Work out the finished part from the listing and answer in its coordinate system (mm). Face numbers are marked on the shaded views. A direction names the side the tool comes from. Coordinates: 2 decimals unless noted, no trailing zeros. Write each loop counter-clockwise with the first axis right and the second up, starting at its lowest first coordinate (ties: lowest second). Pieces come first, ordered by that corner, then holes. Notation, with made-up numbers: (59, 16.5) - (111, 16.5) arc R28 cw to (111, 53.5) - close; hole circle Ø2 at (1.5, -33). An arc over 180 degrees is marked (long way). Use a Markdown table: item, result. Add a question column.
(1) For a pull along Y with two mould halves and no side action, classify the marked faces 6, 7, 8 and 9 as released by +Y, released by -Y, zero draft, split by the parting line, or undercut.
(2) The part is cut by section C-C, the plane y = -9.5. Give the vertices of the cut face in (x, z).
(3) The part is cut by section B-B, the plane x = 0. Give the vertices of the cut face in (y, z), then the cut area to 3 significant figures.
(4) A tool of negligible diameter and unlimited length cuts with its end or side. For the marked faces 1, 2, 3, 4 and 5, from which of +Z, -Z, +X, -X, +Y, -Y can it reach the whole face along a straight path? Write none if from no direction.
(5) The part is cut by section A-A, the plane y = -37. Give the vertices of the cut face in (x, z).
(6) Find the intervals of material crossed by line 1 (Y direction, x = 0, z = 2.25); line 2 (X direction, y = -57, z = 3); line 3 (Y direction, x = 19, z = 7.5), in increasing order. Write a range as from..to.
(7) The part is cut by section D-D, the plane z = 4.25. Give the vertices of the cut face in (x, y).
(8) Given pin 1 Ø10 at (x, y) = (-1, -83) entering from +Z; pin 2 Ø2 at (x, z) = (-22, 3.5) entering from -Y; pin 3 Ø2 at (y, z) = (-29, 8) entering from +X; pin 4 Ø10 at (x, y) = (-3, -54) entering from -Z, each flat-ended and moving along its own axis, determine where each tip first touches the part or whether it passes through.
from build123d import *

# Parameters (mm, degrees)
SKETCH2_R           = 5.08
BOSS_EXTRUDE1_DEPTH = 8.89
CUT_EXTRUDE1_DEPTH  = 8.89
CUT_EXTRUDE4_DEPTH  = 1.778
CUT_EXTRUDE5_START  = -1.778
CUT_EXTRUDE5_DEPTH  = 1.778
SKETCH13_W          = 8.89
SKETCH13_H          = 6.560107066
BOSS_EXTRUDE6_DEPTH = 7.62
SKETCH14_W          = 8.89
SKETCH14_H          = 6.560107066
BOSS_EXTRUDE7_DEPTH = 7.62
FILLET1_R           = 2.032
SKETCH15_R          = 3.556
CUT_EXTRUDE6_DEPTH  = 3.81


with BuildPart() as part:
    # Sketch2 → Boss-Extrude1 (new body)
    with BuildSketch(Plane.XY):
        with BuildLine():
            Line((-10.406791551, -8.202588674), (-10.406791551, -66.622588674))
            ThreePointArc((-10.406791551, -66.622588674), (-12.510019722, -78.309204867), (-18.555768436, -88.529258158))
            Line((-18.555768436, -88.529258158), (-18.555768436, -95.089365224))
            Line((-18.555768436, -95.089365224), (18.555768436, -95.089365224))
            Line((18.555768436, -95.089365224), (18.555768436, -88.529258158))
            ThreePointArc((18.555768436, -88.529258158), (12.510019722, -78.309204867), (10.406791551, -66.622588674))
            Line((10.406791551, -66.622588674), (10.406791551, -8.202588674))
            ThreePointArc((10.406791551, -8.202588674), (0, 0), (-10.406791551, -8.202588674))
        make_face()
        with Locations((0, -10.702948686)):
            Circle(SKETCH2_R, mode=Mode.SUBTRACT)
    extrude(amount=BOSS_EXTRUDE1_DEPTH)

    # Sketch3 → Cut-Extrude1 (cut)
    with BuildSketch(Plane.XY.offset(8.89)):
        with BuildLine():
            Line((-15.392321471, -95.089365224), (15.087678529, -95.089365224))
            ThreePointArc((15.087678529, -95.089365224), (-0.152321471, -79.849365224), (-15.392321471, -95.089365224))
        make_face()
    extrude(amount=-CUT_EXTRUDE1_DEPTH, mode=Mode.SUBTRACT)

    # Sketch8 → Cut-Extrude4 (cut)
    with BuildSketch(Plane.XY.offset(8.89)):
        with BuildLine():
            Line((-6.35, -32.367098726), (-6.35, -57.618798646))
            ThreePointArc((-6.35, -57.618798646), (0, -63.968798646), (6.35, -57.618798646))
            Line((6.35, -57.618798646), (6.35, -32.367098726))
            ThreePointArc((6.35, -32.367098726), (0, -26.017098726), (-6.35, -32.367098726))
        make_face()
    extrude(amount=-CUT_EXTRUDE4_DEPTH, mode=Mode.SUBTRACT)

    # Sketch9 → Cut-Extrude5 (cut)
    with BuildSketch(Plane(origin=(0, 0, 0), x_dir=(-1, 0, 0), z_dir=(0, 0, -1)).offset(CUT_EXTRUDE5_START)):
        with BuildLine():
            Line((6.35, -57.618798646), (6.35, -32.367098726))
            ThreePointArc((6.35, -32.367098726), (0, -26.017098726), (-6.35, -32.367098726))
            Line((-6.35, -32.367098726), (-6.35, -57.618798646))
            ThreePointArc((-6.35, -57.618798646), (0, -63.968798646), (6.35, -57.618798646))
        make_face()
    extrude(amount=CUT_EXTRUDE5_DEPTH, mode=Mode.SUBTRACT)

    # Sketch13 → Boss-Extrude6 (add)
    with BuildSketch(Plane.ZY.offset(18.555768436)):
        with Locations((4.445, -91.809311691)):
            Rectangle(SKETCH13_W, SKETCH13_H)
    extrude(amount=BOSS_EXTRUDE6_DEPTH)

    # Sketch14 → Boss-Extrude7 (add)
    with BuildSketch(Plane(origin=(18.555768436, 0, 0), x_dir=(0, 0, -1), z_dir=(1, 0, 0))):
        with Locations((-4.445, -91.809311691)):
            Rectangle(SKETCH14_W, SKETCH14_H)
    extrude(amount=BOSS_EXTRUDE7_DEPTH)

    # Fillet1
    # the kernel refuses this fillet: 2.032 mm, written as the material it takes off along each edge
    with BuildSketch(Plane(origin=(0, -57.618798646, 0), x_dir=(1, 0, 0), z_dir=(0, 1, 0))) as fillet1_piece_1:
        with BuildLine():
            CenterArc((8.366062499, -2.032), FILLET1_R, 90, 82.819244219)
            Line((6.35, -1.778), (6.30967875, -1.77292))
            ThreePointArc((6.30967875, -1.77292), (6.30936, -0.889), (6.30936, 0))
            Line((6.30936, 0), (6.35, 0.04064))
            Line((6.35, 0.04064), (8.366062499, 0.04064))
            Line((8.366062499, 0.04064), (8.366062499, 0))
        make_face()
    revolve(axis=Axis((0, -57.618798646, 0), (0, 0, -1)), revolution_arc=180, mode=Mode.SUBTRACT)
    with BuildSketch(Plane(origin=(-6.35, -57.618798646, 0), x_dir=(-1, 0, 0), z_dir=(0, 1, 0)), Plane(origin=(6.35, -32.367098726, 0), x_dir=(1, 0, 0), z_dir=(0, -1, 0)), Plane(origin=(-6.35, -32.367098726, 8.89), x_dir=(-1, 0, 0), z_dir=(0, -1, 0)), Plane(origin=(6.35, -57.618798646, 8.89), x_dir=(1, 0, 0), z_dir=(0, 1, 0))) as fillet1_piece_2:
        with BuildLine():
            CenterArc((2.016062499, 2.032), FILLET1_R, 187.180755781, 82.819244219)
            Line((0, 1.778), (-0.04032125, 1.77292))
            ThreePointArc((-0.04032125, 1.77292), (-0.04064, 0.889), (-0.04064, 0))
            Line((-0.04064, 0), (0, -0.04064))
            Line((0, -0.04064), (2.016062499, -0.04064))
            Line((2.016062499, -0.04064), (2.016062499, 0))
        make_face()
    extrude(amount=25.251699921, mode=Mode.SUBTRACT)
    with BuildSketch(Plane(origin=(0, -32.367098726, 0), x_dir=(-1, 0, 0), z_dir=(0, -1, 0))) as fillet1_piece_3:
        with BuildLine():
            CenterArc((8.366062499, -2.032), FILLET1_R, 90, 82.819244219)
            Line((6.35, -1.778), (6.30967875, -1.77292))
            ThreePointArc((6.30967875, -1.77292), (6.30936, -0.889), (6.30936, 0))
            Line((6.30936, 0), (6.35, 0.04064))
            Line((6.35, 0.04064), (8.366062499, 0.04064))
            Line((8.366062499, 0.04064), (8.366062499, 0))
        make_face()
    revolve(axis=Axis((0, -32.367098726, 0), (0, 0, -1)), revolution_arc=180, mode=Mode.SUBTRACT)
    with BuildSketch(Plane(origin=(0, -32.367098726, 8.89), x_dir=(1, 0, 0), z_dir=(0, -1, 0))) as fillet1_piece_4:
        with BuildLine():
            CenterArc((8.366062499, -2.032), FILLET1_R, 90, 82.819244219)
            Line((6.35, -1.778), (6.30967875, -1.77292))
            ThreePointArc((6.30967875, -1.77292), (6.30936, -0.889), (6.30936, 0))
            Line((6.30936, 0), (6.35, 0.04064))
            Line((6.35, 0.04064), (8.366062499, 0.04064))
            Line((8.366062499, 0.04064), (8.366062499, 0))
        make_face()
    revolve(axis=Axis((0, -32.367098726, 8.89), (0, 0, 1)), revolution_arc=180, mode=Mode.SUBTRACT)
    with BuildSketch(Plane(origin=(0, -57.618798646, 8.89), x_dir=(-1, 0, 0), z_dir=(0, 1, 0))) as fillet1_piece_5:
        with BuildLine():
            CenterArc((8.366062499, -2.032), FILLET1_R, 90, 82.819244219)
            Line((6.35, -1.778), (6.30967875, -1.77292))
            ThreePointArc((6.30967875, -1.77292), (6.30936, -0.889), (6.30936, 0))
            Line((6.30936, 0), (6.35, 0.04064))
            Line((6.35, 0.04064), (8.366062499, 0.04064))
            Line((8.366062499, 0.04064), (8.366062499, 0))
        make_face()
    revolve(axis=Axis((0, -57.618798646, 8.89), (0, 0, 1)), revolution_arc=180, mode=Mode.SUBTRACT)

    # Sketch15 → Cut-Extrude6 (cut)
    with BuildSketch(Plane.XZ.offset(95.089365224)):
        with Locations(Location((-20.784044953, 4.445, 0), (0, 0, 270))):
            Circle(SKETCH15_R)
        with Locations(Location((20.479402012, 4.445, 0), (0, 0, 270))):
            Circle(SKETCH15_R)
    extrude(amount=-CUT_EXTRUDE6_DEPTH, mode=Mode.SUBTRACT)


solid = part.part
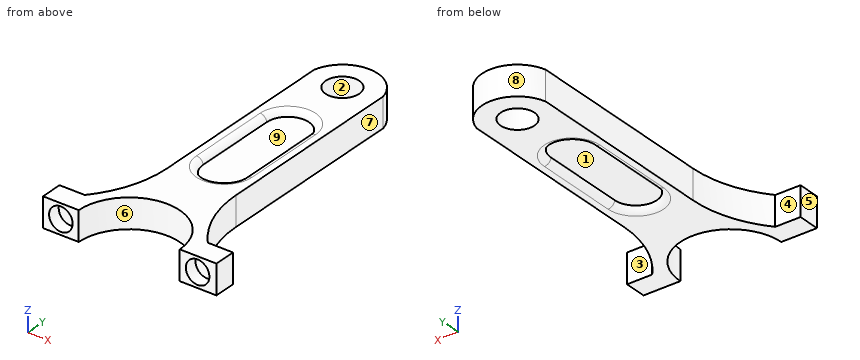
Model answer:
| question | item | result |
|---|---|---|
| 1 | face 6 | released by -Y |
| 1 | face 7 | zero draft |
| 1 | face 8 | released by +Y |
| 1 | face 9 | undercut |
| 2 | outline | (-10.41, 0) - (-4.94, 0) - (-4.94, 8.89) - (-10.41, 8.89) - close; (4.94, 0) - (10.41, 0) - (10.41, 8.89) - (4.94, 8.89) - close |
| 3 | outline | (-79.85, 0) - (-65.98, 0) arc R2.03 ccw to (-63.97, 1.78) - (-26.02, 1.78) arc R2.03 ccw to (-24, 0) - (-15.78, 0) - (-15.78, 8.89) - (-24, 8.89) arc R2.03 ccw to (-26.02, 7.11) - (-63.97, 7.11) arc R2.03 ccw to (-65.98, 8.89) - (-79.85, 8.89) - close; (-5.62, 0) - (0, 0) - (0, 8.89) - (-5.62, 8.89) - close |
| 3 | area | 481 mm^2 |
| 4 | face 1 | -Z |
| 4 | face 2 | +Z, -Z |
| 4 | face 3 | +Z, -Z, +X, +Y |
| 4 | face 4 | +Z, -Z, -X, +Y |
| 4 | face 5 | +Z, -Z, -X, +Y, -Y |
| 5 | outline | (-10.41, 0) - (-8.37, 0) arc R2.03 ccw to (-6.35, 1.78) - (6.35, 1.78) arc R2.03 ccw to (8.37, 0) - (10.41, 0) - (10.41, 8.89) - (8.37, 8.89) arc R2.03 ccw to (6.35, 7.11) - (-6.35, 7.11) arc R2.03 ccw to (-8.37, 8.89) - (-10.41, 8.89) - close |
| 6 | line 1 | -79.85..-15.78, -5.62..0 |
| 6 | line 2 | -10.41..10.41 |
| 6 | line 3 | -91.28..-88.53 |
| 7 | outline | (-26.18, -95.09) - (-24.33, -95.09) - (-24.33, -91.28) - (-17.23, -91.28) - (-17.23, -95.09) - (-15.39, -95.09) arc R15.24 cw to (15.09, -95.09) - (16.93, -95.09) - (16.93, -91.28) - (24.03, -91.28) - (24.03, -95.09) - (26.18, -95.09) - (26.18, -88.53) - (18.56, -88.53) arc R33.52 cw to (10.41, -66.62) - (10.41, -8.2) arc R10.7 ccw to (-10.41, -8.2) - (-10.41, -66.62) arc R33.52 cw to (-18.56, -88.53) - (-26.18, -88.53) - close; hole circle Ø10.16 at (0, -10.7) |
| 8 | pin 1 | z = 8.89 |
| 8 | pin 2 | y = -91.28 |
| 8 | pin 3 | x = 10.41 |
| 8 | pin 4 | z = 0.03 |
